The model under review builds one solid part; all positions refer to its coordinate system, in mm. A direction names the side the tool comes from. Round coordinates to 2 decimals unless told otherwise and drop trailing zeros. Loops run counter-clockwise (first coordinate to the right, second up) from the corner with the lowest first, then second, coordinate; pieces in that order, holes last. Notation, with made-up numbers: M 82.5,34 L 106.5,34 A18 ccw 106.5,56 Z; hole C 36.5,24.25 d5. An arc over 180 degrees is marked long. Answer in a Markdown table with one row per item. Add a question column.
from build123d import *

# Parameters (mm, degrees)
SKETCH1_R           = 4
BOSS_EXTRUDE1_DEPTH = 15
SKETCH2_R           = 1.5
BOSS_EXTRUDE4_DEPTH = 3
FILLET4_R           = 2
SKETCH7_R           = 4
BOSS_EXTRUDE5_DEPTH = 13
SKETCH8_R           = 1.5
CUT_EXTRUDE6_DEPTH  = 10
SKETCH10_R          = 1.25
CUT_EXTRUDE7_DEPTH  = 10
SKETCH11_R          = 2.5
BOSS_EXTRUDE6_DEPTH = 5
SKETCH12_R          = 1.25
CUT_EXTRUDE8_DEPTH  = 5
CUT_EXTRUDE10_START = -1
SKETCH14_R          = 4
CUT_EXTRUDE10_DEPTH = 1


with BuildPart() as part:
    # Sketch1 → Boss-Extrude1 (new body)
    with BuildSketch(Plane(origin=(0, 0, 0), x_dir=(1, 0, 0), z_dir=(0, 1, 0))):
        with Locations(Location((0, 0, 0), (0, 0, 270))):
            Circle(SKETCH1_R)
    extrude(amount=BOSS_EXTRUDE1_DEPTH)

    # Sketch2 → Boss-Extrude4 (add)
    with BuildSketch(Plane(origin=(0, 15, 0), x_dir=(1, 0, 0), z_dir=(0, 1, 0))):
        with BuildLine():
            Line((21.256644483, 1.459786884), (0, 4.5))
            ThreePointArc((0, 4.5), (-4.5, 0), (0, -4.5))
            Line((0, -4.5), (21.256644483, -1.459786884))
            ThreePointArc((21.256644483, -1.459786884), (21.5, 0), (21.256644483, 1.459786884))
        make_face()
        with Locations(Location((18.5, 0, 0), (0, 0, 270))):
            Circle(SKETCH2_R, mode=Mode.SUBTRACT)
    extrude(amount=BOSS_EXTRUDE4_DEPTH)

    # Fillet4
    # the kernel refuses this fillet: 2 mm, written as the material it takes off along each edge
    with BuildSketch(Plane(origin=(21.256644483, 9.943560337, -1.459786884), x_dir=(0.10352186513244716, 0, 0.9946271781122308), z_dir=(0, 1, 0))) as fillet4_piece_1:
        with BuildLine():
            CenterArc((1.573114562, -1.948841845), FILLET4_R, 77.012959975, 88.905549933)
            Line((-0.366786771, -1.462238498), (0, 0))
            ThreePointArc((0, 0), (1.011287933, 0.115105849), (2.022575865, 0))
        make_face()
    extrude(amount=13.112879326, mode=Mode.SUBTRACT)
    with BuildSketch(Plane(origin=(21.256644483, 9.943560337, 1.459786884), x_dir=(-0.9899263374983104, 0, 0.14158335469673372), z_dir=(0, 1, 0))) as fillet4_piece_2:
        with BuildLine():
            CenterArc((1.507539041, -2), FILLET4_R, 90, 88.905549933)
            ThreePointArc((-0.492096093, -1.961798809), (-0.357695041, -0.952893959), (0, 0))
            Line((0, 0), (1.507539041, 0))
        make_face()
    extrude(amount=13.112879326, mode=Mode.SUBTRACT)

    # Sketch7 → Boss-Extrude5 (add)
    with BuildSketch(Plane(origin=(0, 18, 0), x_dir=(1, 0, 0), z_dir=(0, 1, 0))):
        with Locations(Location((0, 0, 0), (0, 0, 270))):
            Circle(SKETCH7_R)
    extrude(amount=BOSS_EXTRUDE5_DEPTH)

    # Sketch8 → Cut-Extrude6 (cut)
    with BuildSketch(Plane(origin=(0, 31, 0), x_dir=(1, 0, 0), z_dir=(0, 1, 0))):
        with Locations(Location((0, 0, 0), (0, 0, 270))):
            Circle(SKETCH8_R)
    extrude(amount=-CUT_EXTRUDE6_DEPTH, mode=Mode.SUBTRACT)

    # Sketch10 → Cut-Extrude7 (cut)
    with BuildSketch(Plane.XZ):
        with Locations(Location((0, 0, 0), (0, 0, 270))):
            Circle(SKETCH10_R)
    extrude(amount=-CUT_EXTRUDE7_DEPTH, mode=Mode.SUBTRACT)

    # Sketch11 → Boss-Extrude6 (add)
    with BuildSketch(Plane.XZ.offset(-15)):
        with Locations(Location((8.5, 0, 0), (0, 0, 90))):
            Circle(SKETCH11_R)
    extrude(amount=BOSS_EXTRUDE6_DEPTH)

    # Sketch12 → Cut-Extrude8 (cut)
    with BuildSketch(Plane.XZ.offset(-10)):
        with Locations(Location((8.5, 0, 0), (0, 0, 270))):
            Circle(SKETCH12_R)
    extrude(amount=-CUT_EXTRUDE8_DEPTH, mode=Mode.SUBTRACT)

    # Sketch14 → Cut-Extrude10 (cut)
    with BuildSketch(Plane(origin=(0, 31, 0), x_dir=(1, 0, 0), z_dir=(0, 1, 0)).offset(CUT_EXTRUDE10_START)):
        with Locations(Location((0, 0, 0), (0, 0, 90))):
            Circle(SKETCH14_R)
    extrude(amount=CUT_EXTRUDE10_DEPTH, mode=Mode.SUBTRACT)


solid = part.part
1. Take a section at C-C, the plane x = 3.25. State the section outline as (y, z) points, and give its area (3 significant figures).
2. Take a section at D-D, the plane z = 3.5. State the section outline as (x, y) points, and give its area (3 significant figures).
3. Mouldability with a two-part tool opening along Z and no side actions: class faces 1 (the cylindrical face through (0.45, 25.56, 1.43)), 2 (the flat face through (1, 0, 1)), 3 (the flat face through (10.02, 16.479, -3.067)) as released by +Z, released by -Z, zero draft, split by the parting line, or undercut.
4. To check wall thickness, follow probe 1 along X at (y, z) = (12.95, 0); probe 2 along X at (y, z) = (25, 0); probe 3 along X at (y, z) = (6.75, 0). State the ranges of each line that lie inside material, in increasing order.
5. Take a section at B-B, the plane x = 18.5. State the section outline as (y, z) points, and give its area (3 significant figures).
6. Machinability: for faces 4 (the flat face through (0, 21, 0)), 5 (the flat face through (0, 10, 0)), 6 (the flat face through (7, 10, 1)), 7 (the cylindrical face through (19.765, 16.479, 0.806)), which of the approach directions +Z, -Z, +X, -X, +Y, -Y give a long, thin tool a straight path to every point of the face, cutting with its end or side? Answer none if there is none.
7. For pin 1 Ø4 at (x, z) = (8.5, 0) entering from -Y; pin 2 Ø5 at (y, z) = (7, -1) entering from -X; pin 3 Ø1.5 at (y, z) = (10.5, -0.5) entering from +X, all flat-tipped, find the tip position at first contact; note any pin that passes through.
8. Take a section at A-A, the plane y = 16.75. State the section outline as (x, z) points.
Check sheet entries:
| question | item | result |
|---|---|---|
| 1 | outline | M 0,-2.33 L 15,-2.33 L 15,-4.04 L 18,-4.04 L 18,-2.33 L 30,-2.33 L 30,2.33 L 18,2.33 L 18,4.04 L 15,4.04 L 15,2.33 L 0,2.33 Z |
| 1 | area | 150 mm^2 |
| 2 | outline | M -2.83,15 L -1.94,15 L -1.94,0 L 1.94,0 L 1.94,15 L 6.99,15 L 6.99,18 L 1.94,18 L 1.94,30 L -1.94,30 L -1.94,18 L -2.83,18 Z |
| 2 | area | 134 mm^2 |
| 3 | face 1 | undercut |
| 3 | face 2 | zero draft |
| 3 | face 3 | released by -Z |
| 4 | probe 1 | x = -4 to 4, 6 to 7.25, 9.75 to 11 |
| 4 | probe 2 | x = -4 to -1.5, 1.5 to 4 |
| 4 | probe 3 | x = -4 to -1.25, 1.25 to 4 |
| 5 | outline | M 15,-1.85 L 18,-1.85 L 18,-1.5 L 15,-1.5 Z; M 15,1.5 L 18,1.5 L 18,1.85 L 15,1.85 Z |
| 5 | area | 2.12 mm^2 |
| 6 | face 4 | +Y |
| 6 | face 5 | -Y |
| 6 | face 6 | +Z, -Z, +X, -Y |
| 6 | face 7 | +Y, -Y |
| 7 | pin 1 | stops at y = 10 |
| 7 | pin 2 | stops at x = -4 |
| 7 | pin 3 | stops at x = 11 |
| 8 | outline | M 0,-4.5 L 19.76,-1.67 A2 ccw 21.46,0 A2 ccw 19.76,1.67 L 0,4.5 A4.5 ccw Z; hole C 18.5,0 d3 |
